Source: CAD feature listing. Evaluate the final solid. Frame: model axes, mm. Face numbers are marked on the shaded views. A direction names the side the tool comes from. Round coordinates to 2 decimals unless told otherwise and drop trailing zeros. Loops run counter-clockwise (first coordinate to the right, second up) from the corner with the lowest first, then second, coordinate; pieces in that order, holes last.
Item 1: Access query for the marked faces 1, 2 and 3. Directions: +Z, -Z, +X, -X, +Y, -Y. A direction counts if a zero-diameter tool reaches every point of the face in a straight line with its end or side. Return the directions, or none.
Item 2: First-contact query: P1, Ø1, axis at x = 46, y = 4.5, coming from the +Z side; P2, Ø2.5, axis at y = 5, z = -28, coming from the -X side; P3, Ø3, axis at y = 0.5, z = -5, coming from the +X side; P4, Ø5.5, axis at y = -1.5, z = -0.5, coming from the -X side. Flat tips, straight axial feed; report the tip coordinate or a pass-through.
Item 3: Section query B-B on x = 5. Return loops of the section in (y, z).
Item 4: Ray query, L1, parallel to X at y = 2.05, z = 0; L2, parallel to X at y = 3.7, z = -20; L3, parallel to Y at x = 35.5, z = -8. Return the intervals inside material, ascending.
Item 5: Pull-direction query (Z, two-part tool) for the marked faces 4, 5 and 6; classes: released by +Z, released by -Z, zero draft, split by the parting line, or undercut.
Item 6: Section query D-D on z = -9. Return loops of the section in (x, y), then the cut area to 3 significant figures.
Item 7: Section query A-A on z = -20. Return loops of the section in (x, y), then the cut area to 4 significant figures.
Item 8: Section query C-C on y = -2.5. Return loops of the section in (x, z).
```python
from build123d import *

# Parameters (mm, degrees)
SKETCH1_W             = 10
SKETCH1_H             = 10
SKETCH1_R             = 4
BOSS_EXTRUDE1_DEPTH   = 5
BOSS_EXTRUDE1_2_DEPTH = 5
SKETCH2_W             = 5
SKETCH2_H             = 10
BOSS_EXTRUDE2_DEPTH   = 5
SKETCH4_W             = 10
SKETCH4_H             = 30
BOSS_EXTRUDE4_DEPTH   = 2.5
BOSS_EXTRUDE7_DEPTH   = 1.5


with BuildPart() as part:
    # Sketch1 → Boss-Extrude1 (new body)
    with BuildSketch(Plane(origin=(0, 0, 0), x_dir=(1, 0, 0), z_dir=(0, 1, 0))):
        with Locations((5, 0)):
            Rectangle(SKETCH1_W, SKETCH1_H)
        with Locations(Location((5, 0, 0), (0, 0, 270))):
            Circle(SKETCH1_R, mode=Mode.SUBTRACT)
    extrude(amount=BOSS_EXTRUDE1_DEPTH)

    # Sketch2 → Boss-Extrude2 (add)
    with BuildSketch(Plane(origin=(10, 0, 0), x_dir=(0, 0, -1), z_dir=(1, 0, 0))):
        Rectangle(SKETCH2_W, SKETCH2_H)
        with Locations((20, 0)):
            Rectangle(SKETCH2_W, SKETCH2_H)
    extrude(amount=BOSS_EXTRUDE2_DEPTH)


with BuildPart() as body_2:
    # Sketch1 → Boss-Extrude1 2 (new body)
    with BuildSketch(Plane(origin=(0, 0, 0), x_dir=(1, 0, 0), z_dir=(0, 1, 0))):
        with Locations((5, 20)):
            Rectangle(SKETCH1_W, SKETCH1_H)
        with Locations(Location((5, 20, 0), (0, 0, 90))):
            Circle(SKETCH1_R, mode=Mode.SUBTRACT)
    extrude(amount=BOSS_EXTRUDE1_2_DEPTH)



with BuildPart() as boss_extrude2_piece_1:
    # of the separate pieces the step leaves, piece 1, a body of its own (boss_extrude2_pieces)
    add(part.part.solids().sort_by_distance((0, 0, -5))[0])

    # Sketch4 → Boss-Extrude4 (add, symmetric)
    with BuildSketch(Plane(origin=(0, 5, 0), x_dir=(1, 0, 0), z_dir=(0, 1, 0))):
        with Locations((15, 10)):
            Rectangle(SKETCH4_W, SKETCH4_H)
    extrude(amount=BOSS_EXTRUDE4_DEPTH, both=True)


with BuildPart() as boss_extrude2_piece_2:
    # of the separate pieces the step leaves, piece 2, a body of its own (boss_extrude2_pieces)
    add(part.part.solids().sort_by_distance((10, -5, -17.5))[0])


with BuildPart() as body_2_1:
    add(body_2.part)

    add(boss_extrude2_piece_1.part)  # Boss-Extrude7 merges Boss-Extrude2 piece 1

    add(boss_extrude2_piece_2.part)  # Boss-Extrude7 merges Boss-Extrude2 piece 2
    # Sketch8 → Boss-Extrude7 (add, symmetric)
    with BuildSketch(Plane(origin=(0, 5, 0), x_dir=(1, 0, 0), z_dir=(0, 1, 0))):
        Polygon((20, 25), (20, 30), (70, 30), (70, 5), (20, -10), (20, -5), (10, -5), (10, 25), align=None)
    extrude(amount=BOSS_EXTRUDE7_DEPTH, both=True)


solid = body_2_1.part
```
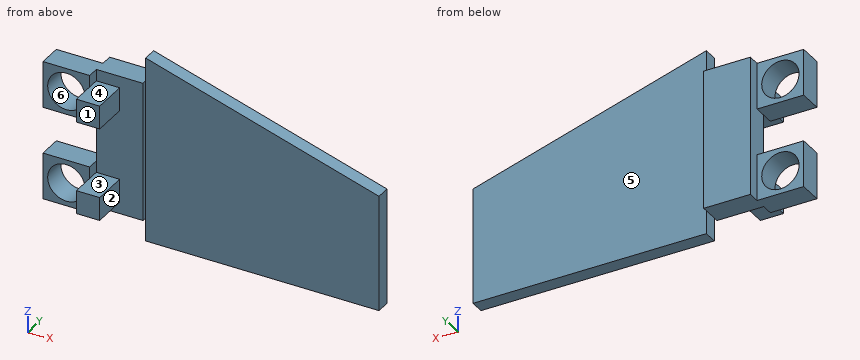
Data:
1. face 1: +Z, -Z, +X, -X, -Y
1. face 2: +Z, -Z, +X, -Y
1. face 3: +X, -Y
2. P1: stops at z = 2.35
2. P2: stops at x = 20
2. P3: stops at x = 10
2. P4: stops at x = 0
3. outline: (0, -25) - (5, -25) - (5, -24) - (0, -24) - close; (0, -16) - (5, -16) - (5, -15) - (0, -15) - close; (0, -5) - (5, -5) - (5, -4) - (0, -4) - close; (0, 4) - (5, 4) - (5, 5) - (0, 5) - close
4. L1: x = 0 to 1, 9 to 15
4. L2: x = 0 to 1, 9 to 70
4. L3: y = 3.5 to 6.5
5. face 4: released by +Z
5. face 5: zero draft
5. face 6: undercut
6. outline: (10, 2.5) - (20, 2.5) - (20, 3.5) - (70, 3.5) - (70, 6.5) - (20, 6.5) - (20, 7.5) - (10, 7.5) - close
6. area: 200 mm2
7. outline: (0, 0) - (1, 0) - (1, 5) - (0, 5) - close; (9, 0) - (10, 0) - (10, -5) - (15, -5) - (15, 2.5) - (20, 2.5) - (20, 3.5) - (70, 3.5) - (70, 6.5) - (20, 6.5) - (20, 7.5) - (10, 7.5) - (10, 5) - (9, 5) - close
7. area: 247.5 mm2
8. outline: (10, -22.5) - (15, -22.5) - (15, -17.5) - (10, -17.5) - close; (10, -2.5) - (15, -2.5) - (15, 2.5) - (10, 2.5) - close
